Check sheet for the drawn part. Datum: minimum x, y, z corner. Units: mm. A direction names the side the tool comes from. Give positions to 0.01 mm unless a question says otherwise; leave off trailing zeros. Write each loop counter-clockwise with the first axis right and the second up, starting at its lowest first coordinate (ties: lowest second). Pieces come first, ordered by that corner, then holes. Notation, with made-up numbers: (39.25, 81.25) - (81.25, 81.25) arc R30 cw to (81.25, 105.25) - close; hole circle Ø10 at (-18, 47). An arc over 180 degrees is marked (long way). One line per question, with ' | ' between items. Start each with the question number.
Q1. Section check B-B on z = 3. Record the boundary of the cut face in (x, y).
Q2. Section check C-C on x = 3. Record the boundary of the cut face in (y, z).
Q3. Thickness scan on L1, parallel to X at y = 51.45, z = 3; L2, parallel to X at y = 38.5, z = 6.25; L3, parallel to Y at x = 7.5, z = 4.5. Record the ranges inside material, lowest first. Write a range as [from, to].
Q4. Set-up check for the marked faces 1 and 2: record each of +Z, -Z, +X, -X, +Y, -Y from which the full face is reachable in a straight line by a thin tool's end or side.
Q5. Section check D-D on y = 23.5. Record the boundary of the cut face in (x, z).
Q6. Section check A-A on x = 7.5. Record the boundary of the cut face in (y, z).
Q7. Gauge pin test, flat ends, axial feed: P1, Ø4.5, axis at x = 3, z = 17, coming from the -Y side; P2, Ø6, axis at y = 21.5, z = 7, coming from the -X side. Record the tip position at first contact, or that the pin passes through.
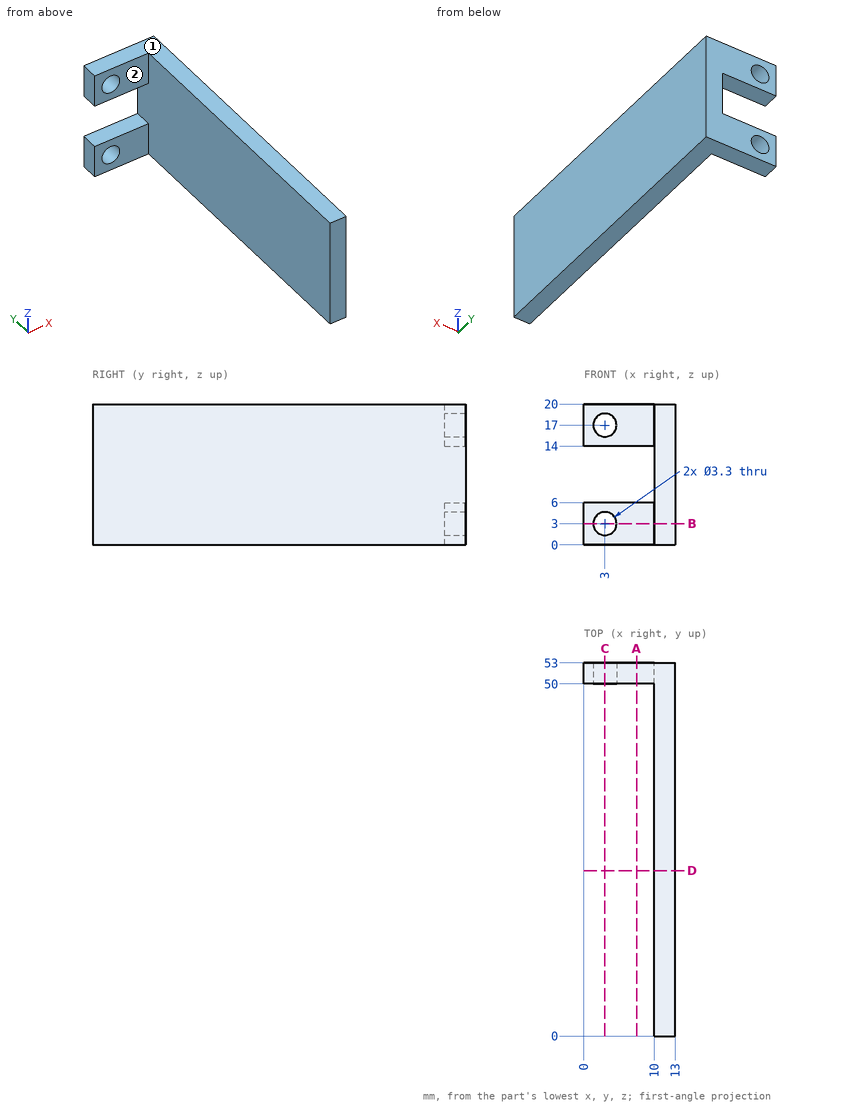
Working result:
1) outline: (0, 50) - (1.35, 50) - (1.35, 53) - (0, 53) - close; (4.65, 50) - (10, 50) - (10, 0) - (13, 0) - (13, 53) - (4.65, 53) - close
2) outline: (50, 0) - (53, 0) - (53, 1.35) - (50, 1.35) - close; (50, 4.65) - (53, 4.65) - (53, 6) - (50, 6) - close; (50, 14) - (53, 14) - (53, 15.35) - (50, 15.35) - close; (50, 18.65) - (53, 18.65) - (53, 20) - (50, 20) - close
3) L1: x = [0, 1.35], [4.65, 13] | L2: x = [10, 13] | L3: y = [50, 53]
4) face 1: +Z, +X, -X, +Y, -Y | face 2: +Z, -Z, -X, -Y
5) outline: (10, 0) - (13, 0) - (13, 20) - (10, 20) - close
6) outline: (50, 0) - (53, 0) - (53, 6) - (50, 6) - close; (50, 14) - (53, 14) - (53, 20) - (50, 20) - close
7) P1: stops at y = 50 | P2: stops at x = 10
